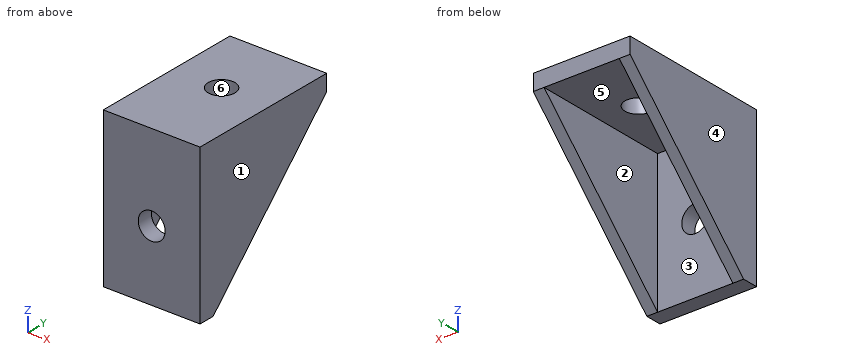
from build123d import *

# Parameters (mm, degrees)
EXTRUDE_THIN1_DEPTH      = 9
EXTRUDE_THIN1_DEPTH_BACK = 9
RIB1_REACH               = 46.788
SKETCH2_WALL_W           = 128.346335328
SKETCH2_WALL_H           = 2
SKETCH3_R                = 2.5
CUT_EXTRUDE1_DEPTH       = 10
SKETCH4_R                = 2.5
CUT_EXTRUDE2_DEPTH       = 10


with BuildPart() as part:
    # Sketch1 → Extrude-Thin1 (new, two sides)
    with BuildSketch(Plane(origin=(0, 0, 0), x_dir=(0, 0, -1), z_dir=(1, 0, 0))) as extrude_thin1_sk:
        Polygon((0, 29), (0, 0), (29, 0), (29, 3), (3, 3), (3, 29), align=None)
    extrude(amount=EXTRUDE_THIN1_DEPTH)
    extrude(extrude_thin1_sk.sketch, amount=-EXTRUDE_THIN1_DEPTH_BACK)

    # Sketch2 wall → Rib1 (add, up to next)
    with BuildSketch(Plane(origin=(9, 16, -16), x_dir=(0, -0.707106781187, -0.707106781187), z_dir=(0, 0.707106781187, -0.707106781187)), mode=Mode.PRIVATE) as rib1_sk1:
        with Locations((0, 1)):
            Rectangle(SKETCH2_WALL_W, SKETCH2_WALL_H)
    rib1_tool1 = extrude(rib1_sk1.sketch, amount=-RIB1_REACH, mode=Mode.PRIVATE) - part.part
    rib1 = rib1_tool1.solids().sort_by_distance((9, 16, -16))[0]
    add(rib1)

    # Mirror1: Rib1 across plane
    add(rib1.mirror(Plane(origin=(0, 0, 0), x_dir=(0, 0, 1), z_dir=(1, 0, 0))))

    # Sketch3 → Cut-Extrude1 (cut)
    with BuildSketch(Plane(origin=(0, 3, 0), x_dir=(1, 0, 0), z_dir=(0, 1, 0))):
        with Locations(Location((0, 16, 0), (0, 0, 270))):
            Circle(SKETCH3_R)
    extrude(amount=-CUT_EXTRUDE1_DEPTH, mode=Mode.SUBTRACT)

    # Sketch4 → Cut-Extrude2 (cut)
    with BuildSketch(Plane(origin=(0, 0, -3), x_dir=(-1, 0, 0), z_dir=(0, 0, -1))):
        with Locations(Location((0, 16, 0), (0, 0, 90))):
            Circle(SKETCH4_R)
    extrude(amount=-CUT_EXTRUDE2_DEPTH, mode=Mode.SUBTRACT)


solid = part.part
Check sheet for the modelled part. Datum: model origin and axes. Units: mm. Face numbers are marked on the shaded views. A direction names the side the tool comes from. Give positions to 0.01 mm unless a question says otherwise; leave off trailing zeros. Order: outer loops, then holes, each group sorted by start corner. A loop starts at its lowest first (then second) coordinate and runs counter-clockwise, first axis right, second up. Notation, with made-up numbers: M -13,4 L 44,4 A25 cw 44,42 Z; hole C 69.5,2 d2. An arc over 180 degrees is marked long. Answer as CSV lines item,"result". Start each with the question number.
Item 1: Gauge pin test, flat ends, axial feed: P1, Ø8, axis at x = 0, z = -16, coming from the +Y side; P2, Ø4.5, axis at x = 0, y = 16, coming from the -Z side; P3, Ø4, axis at x = 2, y = 11.5, coming from the -Z side; P4, Ø10, axis at x = 4, z = -9, coming from the +Y side. Record the tip position at first contact, or that the pin passes through.
Item 2: Tool access check on the marked faces 5 and 6. Record the directions out of +Z, -Z, +X, -X, +Y, -Y that give a thin tool (end or side, any length) a straight path to the whole face; none if there is none.
Item 3: Cross-section at D-D on y = 8.75. Enter the section's corners in (x, z), plus the area to 3 significant figures.
Item 4: Thickness scan on line 1 (X direction, y = 11.5, z = -8.25); line 2 (X direction, y = 1.8, z = -16); line 3 (Y direction, x = -3.25, z = -11). Record the ranges inside material, lowest first. Write a range as [from, to].
Item 5: Cross-section at C-C on z = -16. Enter the section's corners in (x, y).
Item 6: Mould release check, pull along X, two halves, no side actions. Record for the marked faces 1, 2, 3 and 4: +X half, -X half, draft (parallel to the pull), parting line (faces both ways), or undercut.
Item 7: Cross-section at B-B on x = 0. Enter the section's corners in (y, z), plus the area to 3 significant figures.
Item 8: Cross-section at A-A on y = 16. Enter the section's corners in (x, z).
Established:
1,P1,"stops at y = 3"
1,P2,"passes through"
1,P3,"stops at z = -3"
1,P4,"stops at y = 27"
2,face 5,"-Z, +Y"
2,face 6,"+Z, -Z"
3,outline,"M -9,-23.25 L -7,-23.25 L -7,-3 L 7,-3 L 7,-23.25 L 9,-23.25 L 9,0 L -9,0 Z"
3,area,"135 mm^2"
4,line 1,"x = [-9, -7], [7, 9]"
4,line 2,"x = [-9, -2.5], [2.5, 9]"
4,line 3,"y = [0, 3]"
5,outline,"M -9,0 L -2.5,0 L -2.5,3 L -7,3 L -7,16 L -9,16 Z; M 2.5,0 L 9,0 L 9,16 L 7,16 L 7,3 L 2.5,3 Z"
6,face 1,"+X half"
6,face 2,"undercut"
6,face 3,"undercut"
6,face 4,"-X half"
7,outline,"M 0,-29 L 3,-29 L 3,-18.5 L 0,-18.5 Z; M 0,-13.5 L 3,-13.5 L 3,-3 L 13.5,-3 L 13.5,0 L 0,0 Z; M 18.5,-3 L 29,-3 L 29,0 L 18.5,0 Z"
7,area,"135 mm^2"
8,outline,"M -9,-16 L -7,-16 L -7,-3 L -2.5,-3 L -2.5,0 L -9,0 Z; M 2.5,-3 L 7,-3 L 7,-16 L 9,-16 L 9,0 L 2.5,0 Z"
